Build history of the part. All positions in model axes, mm. Face numbers are marked on the shaded views. Give positions to 0.01 mm unless a question says otherwise; leave off trailing zeros. Loops run counter-clockwise (first coordinate to the right, second up) from the corner with the lowest first, then second, coordinate; pieces in that order, holes last. Notation, with made-up numbers: (-3.5, 86.5) -> (2.5, 86.5) arc R17 cw to (2.5, 106.5) -> close; hole circle Ø2 at (42.5, 71). An arc over 180 degrees is marked (long way). Answer in a Markdown table with one row per item. Add a question column.
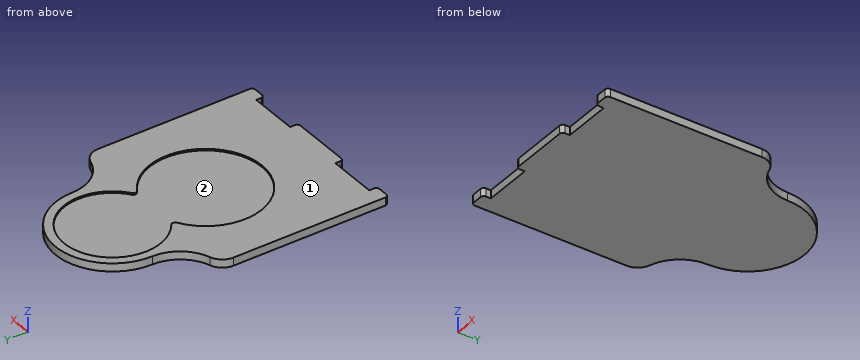
from build123d import *

# Parameters (mm, degrees)
F1_DEPTH = 6.35
F2_R     = 12.7
F3_R     = 2.54
F5_DEPTH = 1.27
F6_R     = 2.54


# Not quite as in the source:
# - a feature names something its author has since deleted; it is built from what else it names


with BuildPart() as f1:
    # F0 (on Top) → F1 (new body)
    with BuildSketch(Plane.XY):
        with BuildLine():
            Line((0, 127), (0, 0))
            Line((0, 0), (0, -6.35))
            Line((0, -6.35), (12.7, -6.35))
            Line((12.7, -6.35), (12.7, 0))
            Line((12.7, 0), (50.8, 0))
            Line((50.8, 0), (50.8, -6.35))
            Line((50.8, -6.35), (101.6, -6.35))
            Line((101.6, -6.35), (101.6, 0))
            Line((101.6, 0), (139.7, 0))
            Line((139.7, 0), (139.7, -6.35))
            Line((139.7, -6.35), (152.4, -6.35))
            Line((152.4, -6.35), (152.4, 0))
            Line((152.4, 0), (152.4, 127))
            ThreePointArc((152.4, 127), (130.249490442, 136.1750414724), (121.0744489697, 158.3255510303))
            ThreePointArc((121.0744489697, 158.3255510303), (76.2, 203.2), (31.3255510303, 158.3255510303))
            ThreePointArc((31.3255510303, 158.3255510303), (22.150509558, 136.1750414724), (0, 127))
        make_face()
    extrude(amount=F1_DEPTH)

    # F2
    f2_edges = [f1.edges().sort_by_distance(p)[0] for p in [
        (0, 127, 3.175),
        (152.4, 127, 3.175),
    ]]
    fillet(f2_edges, radius=F2_R)

    # F3
    f3_edges = [f1.edges().sort_by_distance(p)[0] for p in [
        (0, -6.35, 3.175),
        (12.7, -6.35, 3.175),
        (50.8, -6.35, 3.175),
        (101.6, -6.35, 3.175),
        (139.7, -6.35, 3.175),
        (152.4, -6.35, 3.175),
    ]]
    fillet(f3_edges, radius=F3_R)

    # F4 (on face) → F5 (cut)
    with BuildSketch(Plane.XY.offset(6.35)):
        with BuildLine():
            ThreePointArc((94.7584962883, 125.0510530549), (109.0533766041, 139.0313641932), (114.3, 158.3255510303))
            ThreePointArc((114.3, 158.3255510303), (56.9058131628, 191.1789276345), (57.6415037117, 125.0510530549))
            ThreePointArc((57.6415037117, 125.0510530549), (76.2, 129.1106492996), (94.7584962883, 125.0510530549))
        make_face()
        with BuildLine():
            ThreePointArc((94.7584962883, 125.0510530549), (76.2, 120.2255510303), (57.6415037117, 125.0510530549))
            ThreePointArc((57.6415037117, 125.0510530549), (52.2116972257, 47.2392138647), (120.65, 84.6606492996))
            ThreePointArc((120.65, 84.6606492996), (113.6214354349, 108.6489520739), (94.7584962883, 125.0510530549))
        make_face()
        with BuildLine():
            ThreePointArc((94.7584962883, 125.0510530549), (76.2, 129.1106492996), (57.6415037117, 125.0510530549))
            ThreePointArc((57.6415037117, 125.0510530549), (76.2, 120.2255510303), (94.7584962883, 125.0510530549))
        make_face()
    extrude(amount=-F5_DEPTH, mode=Mode.SUBTRACT)

    # F6
    f6_edges = [f1.edges().sort_by_distance(p)[0] for p in [
        (57.641504, 125.051053, 5.715),
        (94.758496, 125.051053, 5.715),
    ]]
    fillet(f6_edges, radius=F6_R)


solid = f1.part
(1) Saw through at B-B, the plane x = 48.5. List the corners of the cut face in (y, z), then the cut area to 3 significant figures.
(2) Wall check: line 1 along Y through (x, z) = (76.2, 5.55); line 2 along X through (y, z) = (158.5, 3.25); line 3 along X through (y, z) = (192.5, 5.5). Give the ranges that are in metal, low to high. Write a range as from..to.
(3) Saw through at D-D, the plane x = 76.2. List the corners of the cut face in (y, z).
(4) Saw through at C-C, the plane y = 180.5. List the corners of the cut face in (x, z), then the cut area to 3 significant figures.
(5) Two-plate mould, pull along X, no slides. Class the marked faces 1 and 2: released by +X, released by -X, zero draft, split by the parting line, or undercut.
(6) Flat gauge pins, fed straight in: pin 1 Ø1.5 at (x, z) = (96, 1.5) entering from +Y; pin 2 Ø1.9 at (x, z) = (33, 3.5) entering from -Y; pin 3 Ø6 at (x, y) = (79, 95) entering from +Z. Where does each tip first touch, or does it go through?
(7) Saw through at A-A, the plane z = 3. List the corners of the cut face in (x, y).
Worked answers:
| question | item | result |
|---|---|---|
| 1 | outline | (0, 0) -> (193.63, 0) -> (193.63, 6.35) -> (184.49, 6.35) -> (184.49, 5.08) -> (132.17, 5.08) -> (132.17, 6.35) -> (119.42, 6.35) -> (119.42, 5.08) -> (49.9, 5.08) -> (49.9, 6.35) -> (0, 6.35) -> close |
| 1 | area | 1,070 mm^2 |
| 2 | line 1 | -6.35..40.21, 196.43..203.2 |
| 2 | line 2 | 31.33..121.07 |
| 2 | line 3 | 47.12..59.36, 93.04..105.28 |
| 3 | outline | (-6.35, 0) -> (203.2, 0) -> (203.2, 6.35) -> (196.43, 6.35) -> (196.43, 5.08) -> (40.21, 5.08) -> (40.21, 6.35) -> (-6.35, 6.35) -> close |
| 4 | outline | (37.19, 0) -> (115.21, 0) -> (115.21, 6.35) -> (107.18, 6.35) -> (107.18, 5.08) -> (45.22, 5.08) -> (45.22, 6.35) -> (37.19, 6.35) -> close |
| 4 | area | 417 mm^2 |
| 5 | face 1 | zero draft |
| 5 | face 2 | undercut |
| 6 | pin 1 | y = 198.96 |
| 6 | pin 2 | y = 0 |
| 6 | pin 3 | z = 5.08 |
| 7 | outline | (0, -3.81) arc R2.54 ccw to (2.54, -6.35) -> (10.16, -6.35) arc R2.54 ccw to (12.7, -3.81) -> (12.7, 0) -> (50.8, 0) -> (50.8, -3.81) arc R2.54 ccw to (53.34, -6.35) -> (99.06, -6.35) arc R2.54 ccw to (101.6, -3.81) -> (101.6, 0) -> (139.7, 0) -> (139.7, -3.81) arc R2.54 ccw to (142.24, -6.35) -> (149.86, -6.35) arc R2.54 ccw to (152.4, -3.81) -> (152.4, 116.17) arc R12.7 ccw to (143.36, 128.33) arc R31.33 cw to (121.07, 158.33) arc R44.87 ccw to (31.33, 158.33) arc R31.33 cw to (9.04, 128.33) arc R12.7 ccw to (0, 116.17) -> close |
